The drawing under review shows one solid part. Ordinate dimensions are in mm from its lowest x, y, z. Coordinates: 2 decimals unless noted, no trailing zeros. Loops run counter-clockwise (first coordinate to the right, second up) from the corner with the lowest first, then second, coordinate; pieces in that order, holes last. Notation, with made-up numbers: M 62.5,34 L 105.5,34 A36 cw 105.5,73 Z; hole C 84.5,33.5 d5. An arc over 180 degrees is marked long. Put each result on its own line as item: value.
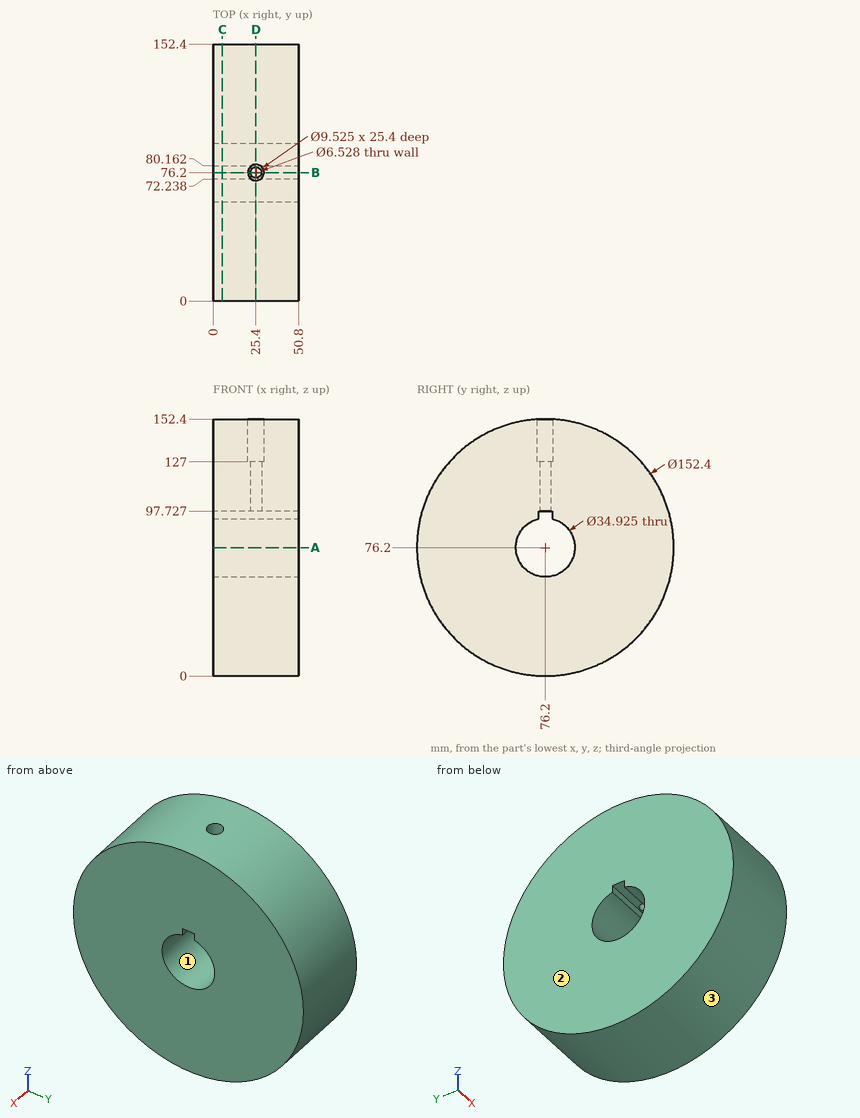
(1) Add section B-B (y = 76.2). Write out the cut boundary in (x, z).
Determined:
outline: M 0,0 L 50.8,0 L 50.8,58.74 L 0,58.74 Z; M 0,97.73 L 22.14,97.73 L 22.14,127 L 20.64,127 L 20.64,152.4 L 0,152.4 Z; M 28.66,97.73 L 50.8,97.73 L 50.8,152.4 L 30.16,152.4 L 30.16,127 L 28.66,127 Z
(2) For pin 1 (5 mm diameter, centred on x = 18, z = 110.5, fed in from -Y); pin 2 (2.5 mm diameter, centred on x = 26.5, z = 95, fed in from +Y); pin 3 (4 mm diameter, centred on x = 45, z = 51.5, fed in from -Y), all flat-tipped, find the tip position at first contact; note any pin that passes through.
Determined:
pin 1: stops at y = 6.95
pin 2: stops at y = 150.35
pin 3: stops at y = 3.46
(3) Add section D-D (x = 25.4). Write out the cut boundary in (y, z) (1 decimal), plus the area to 3 significant figures.
Determined:
outline: M 71.4,127 L 71.4,152.3 A76.2 ccw long 81,152.3 L 81,127 L 79.5,127 L 79.5,97.7 L 80.2,97.7 L 80.2,93.2 A17.5 cw long 72.2,93.2 L 72.2,97.7 L 72.9,97.7 L 72.9,127 Z
area: 16,800 mm^2
(4) Draft analysis for pull direction Z (two halves, no side actions). For the marked faces 1, 2 and 3, state which applies: +Z half, -Z half, draft (parallel to the pull), parting line (faces both ways), or undercut.
Determined:
face 1: undercut
face 2: draft
face 3: parting line
(5) Add section C-C (x = 5.5). Write out the cut boundary in (y, z) (1 decimal), plus the area to 4 significant figures.
Determined:
outline: C 76.2,76.2 d152.4; hole M 72.2,93.2 A17.5 ccw long 80.2,93.2 L 80.2,97.7 L 72.2,97.7 Z
area: 17,250 mm^2
(6) Add section A-A (z = 76.2). Write out the cut boundary in (x, y).
Determined:
outline: M 0,0 L 50.8,0 L 50.8,58.74 L 0,58.74 Z; M 0,93.66 L 50.8,93.66 L 50.8,152.4 L 0,152.4 Z
(7) Wall thickness on line 1 along Z through (x, y) = (36, 76.2); line 2 along X through (y, z) = (76, 110); line 3 along Z through (x, y) = (5, 69.5) (1 decimal): over which ranges is each line inside the solid? List them lowest first. Write a range as [from, to].
Determined:
line 1: z = [0, 58.74], [97.73, 152.4]
line 2: x = [0, 22.14], [28.66, 50.8]
line 3: z = [0.3, 60.1], [92.3, 152.1]
